Could you check a few things on this model? Use its own coordinates, in mm. Face numbers are marked on the shaded views. A direction names the side the tool comes from. Give positions to 0.01 mm unless a question says otherwise; leave off trailing zeros. Loops run counter-clockwise (first coordinate to the right, second up) from the corner with the lowest first, then second, coordinate; pieces in that order, holes last. Notation, with made-up numbers: M -14,52 L 26,52 A31 cw 26,89 Z; hole C -26.5,-15.75 d1. An arc over 180 degrees is marked long. Use a Markdown table: item, result. Add a question column.
1) We'd pull the mould along X, two halves only. Please class the marked faces 1, 2 and 3: +X half, -X half, draft (parallel to the pull), parting line (faces both ways), or undercut.
2) Suppose I cut it at A-A on z = 5. List the corners of the cut face in (x, y) for me, and give its area (3 significant figures).
3) If I drill on line 1 along Z through (x, y) = (-1.55, 0); line 2 along X through (y, z) = (-2.25, 2.5); line 3 along Y through (x, z) = (0.25, 12), over which ranges is the centre line in solid material (lowest first)? Write a range as [from, to].
4) Suppose I cut it at C-C on z = 9.5. List the corners of the cut face in (x, y) for me.
5) Suppose I cut it at D-D on y = -2.25. Count the separate pieces of the cut face and the enclosed holes in it, and give its area (3 significant figures).
6) Suppose I cut it at B-B on y = 0. List the corners of the cut face in (x, z) for me.
7) Will these pins go through, and if not, where does the flat tip stop? pin 1 Ø4 at (y, z) = (0, 5) entering from -X; pin 2 Ø4 at (y, z) = (0, 5) entering from +X; pin 3 Ø5 at (y, z) = (3, 27) entering from -X.
8) Which directions (+Z, -Z, +X, -X, +Y, -Y) give clear straight access to the entire face, cutting with the end or side of a thin tool? Please do the marked faces 4 and 5.
```python
from build123d import *

# Parameters (mm, degrees)
F0_R           = 8
F1_DEPTH       = 34
F3_DEPTH       = 100
F5_DEPTH       = 8.0010001
F5_DEPTH_BACK  = 50
F7_SIZE2       = 1
F7_SIZE        = 1
F8_R           = 1.5
F9_DEPTH       = 50
F9_DEPTH_BACK  = 50
F11_DEPTH      = 50
F11_DEPTH_BACK = 50
F12_R          = 3
F13_DEPTH      = 12
F15_DEPTH      = 10
F17_DEPTH      = 10


with BuildPart() as f1:
    # F0 (on Top) → F1 (new body)
    with BuildSketch(Plane.XY):
        Circle(F0_R)
    extrude(amount=F1_DEPTH)

    # F2 (on Right) → F3 (cut)
    with BuildSketch(Plane.YZ):
        with BuildLine():
            ThreePointArc((4.5470095179, 22.0663473532), (0, 26.613356871), (-4.5470095179, 22.0663473532))
            Line((-4.5470095179, 22.0663473532), (4.5470095179, 22.0663473532))
        make_face()
        with BuildLine():
            Line((4.5470095179, 22.0663473532), (-4.5470095179, 22.0663473532))
            ThreePointArc((-4.5470095179, 22.0663473532), (0, 17.5193378353), (4.5470095179, 22.0663473532))
        make_face()
    extrude(amount=-F3_DEPTH, mode=Mode.SUBTRACT)

    # F4 (on Right) → F5 (cut, two sides)
    with BuildSketch(Plane.YZ) as f5_sk:
        with BuildLine():
            ThreePointArc((5.006999059, 21.9850950465), (-0.093000941, 27.0850950465), (-5.193000941, 21.9850950465))
            Line((-5.193000941, 21.9850950465), (5.006999059, 21.9850950465))
        make_face()
        with BuildLine():
            Line((5.006999059, 21.9850950465), (-5.193000941, 21.9850950465))
            ThreePointArc((-5.193000941, 21.9850950465), (-0.093000941, 16.8850950465), (5.006999059, 21.9850950465))
        make_face()
    extrude(amount=F5_DEPTH, mode=Mode.SUBTRACT)
    extrude(f5_sk.sketch, amount=-F5_DEPTH_BACK, mode=Mode.SUBTRACT)

    # F7
    f7_edges = [f1.edges().sort_by_distance(p)[0] for p in [
        (-8, 0, 34),
    ]]
    chamfer(f7_edges, length=F7_SIZE, length2=F7_SIZE2)

    # F8 (on Right) → F9 (cut, two sides)
    with BuildSketch(Plane.YZ) as f9_sk:
        with Locations((0, 5)):
            Circle(F8_R)
    extrude(amount=-F9_DEPTH, mode=Mode.SUBTRACT)
    extrude(f9_sk.sketch, amount=F9_DEPTH_BACK, mode=Mode.SUBTRACT)

    # F10 (on Right) → F11 (cut, two sides)
    with BuildSketch(Plane.YZ) as f11_sk:
        Polygon((8.5644535553, 4.3144535553), (4.25, 0), (8.5644535553, 0), align=None)
        Polygon((-8.5644535553, 4.3144535553), (-8.5644535553, 0), (-4.25, 0), align=None)
    extrude(amount=-F11_DEPTH, mode=Mode.SUBTRACT)
    extrude(f11_sk.sketch, amount=F11_DEPTH_BACK, mode=Mode.SUBTRACT)

    # F12 (on face) → F13 (cut)
    with BuildSketch(Plane.XY.offset(34)):
        Circle(F12_R)
    extrude(amount=-F13_DEPTH, mode=Mode.SUBTRACT)

    # F14 (on face) → F15 (cut)
    with BuildSketch(Plane.XY.offset(34)):
        Polygon((-4.25, -8.8976696134), (-4.25, 0), (-4.25, 8.1088971347), (-12.2155025601, 8.1088971347), (-12.2155025601, -9.0591032058), align=None)
        Polygon((4.25, 8.1645697355), (4.25, 0), (4.25, -8.8976696134), (9.4557348639, -8.8976696134), (9.4557348639, 8.1645697355), align=None)
    extrude(amount=F15_DEPTH, mode=Mode.SUBTRACT)

    # F16 (on Top) → F17 (cut)
    with BuildSketch(Plane.XY):
        Polygon((-8.8066291064, -8.1897312775), (-4.0295359638, -8.1897312775), (-4.0295359638, 0), (-4.0295359638, 8.8079171255), (-8.8066291064, 8.8079171255), align=None)
        Polygon((4.1875811294, 0), (4.1875811294, -9.2414822429), (9.3784797937, -9.2414822429), (9.3784797937, 8.8079171255), (4.1875811294, 8.8079171255), align=None)
    extrude(amount=F17_DEPTH, mode=Mode.SUBTRACT)


solid = f1.part
```
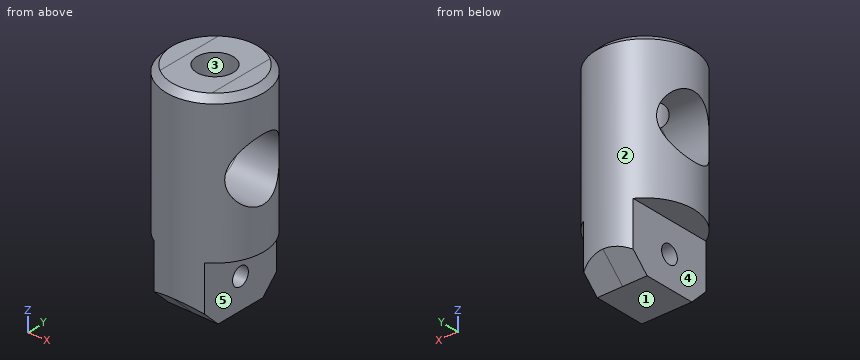
Answer block:
| question | item | result |
|---|---|---|
| 1 | face 1 | draft |
| 1 | face 2 | parting line |
| 1 | face 3 | undercut |
| 2 | outline | M -4.03,-6.91 A8 ccw 4.19,-6.82 L 4.19,-1.5 L -4.03,-1.5 Z; M -4.03,1.5 L 4.19,1.5 L 4.19,6.82 A8 ccw -4.03,6.91 Z |
| 2 | area | 101 mm^2 |
| 3 | line 1 | z = [0, 3.5], [6.5, 16.89] |
| 3 | line 2 | x = [-4.03, 4.19] |
| 3 | line 3 | y = [-8, 8] |
| 4 | outline | M -4.03,-6.91 A8 ccw 4.19,-6.82 L 4.19,6.82 A8 ccw -4.03,6.91 Z |
| 5 | separate pieces | 3 |
| 5 | enclosed holes | 0 |
| 5 | area | 278 mm^2 |
| 6 | outline | M -8,10 L -4.03,10 L -4.03,6.5 L 4.19,6.5 L 4.19,10 L 8,10 L 8,16.89 L -8,16.89 Z; M -8,27.08 L -3,27.08 L -3,34 L -7,34 L -8,33 Z; M -4.03,0 L 4.19,0 L 4.19,3.5 L -4.03,3.5 Z; M 3,27.08 L 8,27.08 L 8,33 L 7,34 L 3,34 Z |
| 7 | pin 1 | stops at x = -4.03 |
| 7 | pin 2 | stops at x = 4.19 |
| 7 | pin 3 | stops at x = -7.98 |
| 8 | face 4 | -Z, -X, +Y, -Y |
| 8 | face 5 | -Z, +X, +Y, -Y |
